For this review, take the finished solid that the model builds, in its own axes (mm). Coordinates: 2 decimals unless noted, no trailing zeros. Loops run counter-clockwise (first coordinate to the right, second up) from the corner with the lowest first, then second, coordinate; pieces in that order, holes last. Notation, with made-up numbers: (33.25, -39) - (90.25, -39) arc R18 cw to (90.25, -28) - close; hole circle Ø10 at (79, 58). An arc over 180 degrees is marked (long way). Answer as a JSON object with one key per item and string values. Group by question number.
Item 1: To check wall thickness, follow line 1 (X direction, y = 1.55, z = -45); line 2 (X direction, y = 1.4, z = 15); line 3 (Z direction, x = -20, y = 0.65). State the ranges of each line that lie inside material, in increasing order.
Item 2: Clearance check with a flat-ended pin moving along its axis: pin 1 (1.5 mm diameter, centred on y = 2.5, z = -92.5, fed in from +X). State where the tip first meets the part, or that it passes through.
Item 3: We need section B-B (z = -15). Give the boundary of the cut face in (x, y).
Item 4: We need section A-A (z = -45). Give the boundary of the cut face in (x, y), then the cut area to 3 significant figures.
Item 5: We need section D-D (y = 0.45). State how many separate pieces and enclosed holes the cut face has, then the cut area to 3 significant figures.
Item 6: We need section C-C (x = -26.5). Give the boundary of the cut face in (y, z).
Item 7: Mouldability with a two-part tool opening along X and no side actions: class faces 1 (the flat face through (-1, 0, -31)), 2 (the cylindrical face through (48.831, 1.521, 14.474)), 3 (the cylindrical face through (1.319, 1.479, -119.985)), 4 (the cylindrical face through (-57.15, 1.52, 56.99)) as released by +X, released by -X, zero draft, split by the parting line, or undercut.
from build123d import *

# Parameters (mm, degrees)
BOSS_EXTRUDE3_DEPTH = 3
FILLET3_R           = 10
SKETCH4_R           = 1.75
CUT_EXTRUDE1_DEPTH  = 3
CUT_EXTRUDE2_REACH  = 5
SKETCH5_R           = 1.75
CUT_EXTRUDE3_REACH  = 5
SKETCH6_R           = 1.5


with BuildPart() as part:
    # Sketch1 → Boss-Extrude3 (new body)
    with BuildSketch(Plane(origin=(0, 0, 0), x_dir=(1, 0, 0), z_dir=(0, 1, 0))):
        with BuildLine():
            Line((-60, 60), (-60, -60))
            Line((-60, -60), (60, -60))
            Line((60, -60), (60, 60))
            ThreePointArc((60, 60), (0, 120), (-60, 60))
        make_face()
    extrude(amount=BOSS_EXTRUDE3_DEPTH)

    # Fillet3
    fillet3_edges = [part.edges().sort_by_distance(p)[0] for p in [
        (60, 1.5, 60),
        (-60, 1.5, 60),
    ]]
    fillet(fillet3_edges, radius=FILLET3_R)

    # Sketch4 → Cut-Extrude1 (cut)
    with BuildSketch(Plane(origin=(0, 3, 0), x_dir=(1, 0, 0), z_dir=(0, 1, 0))):
        with Locations((-26.5, -15)):
            Circle(SKETCH4_R)
        with Locations((-50.5, -15)):
            Circle(SKETCH4_R)
        with Locations((-50.5, 15)):
            Circle(SKETCH4_R)
        with Locations((-26.5, 15)):
            Circle(SKETCH4_R)
    cut_extrude1 = extrude(amount=-CUT_EXTRUDE1_DEPTH, mode=Mode.SUBTRACT)

    # Mirror1: Cut-Extrude1 across plane
    add(cut_extrude1.mirror(Plane(origin=(0, 0, 0), x_dir=(0, 0, 1), z_dir=(1, 0, 0))), mode=Mode.SUBTRACT)

    # Sketch5 → Cut-Extrude2 (cut, up to next)
    with BuildSketch(Plane(origin=(0, 3, 0), x_dir=(1, 0, 0), z_dir=(0, 1, 0)), mode=Mode.PRIVATE) as cut_extrude2_sk1:
        with Locations((20, 75)):
            Circle(SKETCH5_R)
    cut_extrude2_tool1 = extrude(cut_extrude2_sk1.sketch, amount=-CUT_EXTRUDE2_REACH, mode=Mode.PRIVATE) & part.part
    add(cut_extrude2_tool1.solids().sort_by_distance((20, 3, -75))[0], mode=Mode.SUBTRACT)
    # Sketch5 → Cut-Extrude2 (cut, up to next)
    with BuildSketch(Plane(origin=(0, 3, 0), x_dir=(1, 0, 0), z_dir=(0, 1, 0)), mode=Mode.PRIVATE) as cut_extrude2_sk2:
        with Locations((-20, 75)):
            Circle(SKETCH5_R)
    cut_extrude2_tool2 = extrude(cut_extrude2_sk2.sketch, amount=-CUT_EXTRUDE2_REACH, mode=Mode.PRIVATE) & part.part
    add(cut_extrude2_tool2.solids().sort_by_distance((-20, 3, -75))[0], mode=Mode.SUBTRACT)
    # Sketch5 → Cut-Extrude2 (cut, up to next)
    with BuildSketch(Plane(origin=(0, 3, 0), x_dir=(1, 0, 0), z_dir=(0, 1, 0)), mode=Mode.PRIVATE) as cut_extrude2_sk3:
        with Locations((-20, 45)):
            Circle(SKETCH5_R)
    cut_extrude2_tool3 = extrude(cut_extrude2_sk3.sketch, amount=-CUT_EXTRUDE2_REACH, mode=Mode.PRIVATE) & part.part
    add(cut_extrude2_tool3.solids().sort_by_distance((-20, 3, -45))[0], mode=Mode.SUBTRACT)
    # Sketch5 → Cut-Extrude2 (cut, up to next)
    with BuildSketch(Plane(origin=(0, 3, 0), x_dir=(1, 0, 0), z_dir=(0, 1, 0)), mode=Mode.PRIVATE) as cut_extrude2_sk4:
        with Locations((20, 45)):
            Circle(SKETCH5_R)
    cut_extrude2_tool4 = extrude(cut_extrude2_sk4.sketch, amount=-CUT_EXTRUDE2_REACH, mode=Mode.PRIVATE) & part.part
    add(cut_extrude2_tool4.solids().sort_by_distance((20, 3, -45))[0], mode=Mode.SUBTRACT)

    # Sketch6 → Cut-Extrude3 (cut, up to next)
    with BuildSketch(Plane(origin=(0, 3, 0), x_dir=(1, 0, 0), z_dir=(0, 1, 0)), mode=Mode.PRIVATE) as cut_extrude3_sk1:
        with Locations((-38.213203436, 75.786796564)):
            Circle(SKETCH6_R)
    cut_extrude3_tool1 = extrude(cut_extrude3_sk1.sketch, amount=-CUT_EXTRUDE3_REACH, mode=Mode.PRIVATE) & part.part
    add(cut_extrude3_tool1.solids().sort_by_distance((-38.213203, 3, -75.786797))[0], mode=Mode.SUBTRACT)
    # Sketch6 → Cut-Extrude3 (cut, up to next)
    with BuildSketch(Plane(origin=(0, 3, 0), x_dir=(1, 0, 0), z_dir=(0, 1, 0)), mode=Mode.PRIVATE) as cut_extrude3_sk2:
        with Locations((-17, 97)):
            Circle(SKETCH6_R)
    cut_extrude3_tool2 = extrude(cut_extrude3_sk2.sketch, amount=-CUT_EXTRUDE3_REACH, mode=Mode.PRIVATE) & part.part
    add(cut_extrude3_tool2.solids().sort_by_distance((-17, 3, -97))[0], mode=Mode.SUBTRACT)
    # Sketch6 → Cut-Extrude3 (cut, up to next)
    with BuildSketch(Plane(origin=(0, 3, 0), x_dir=(1, 0, 0), z_dir=(0, 1, 0)), mode=Mode.PRIVATE) as cut_extrude3_sk3:
        with Locations((17, 97)):
            Circle(SKETCH6_R)
    cut_extrude3_tool3 = extrude(cut_extrude3_sk3.sketch, amount=-CUT_EXTRUDE3_REACH, mode=Mode.PRIVATE) & part.part
    add(cut_extrude3_tool3.solids().sort_by_distance((17, 3, -97))[0], mode=Mode.SUBTRACT)
    # Sketch6 → Cut-Extrude3 (cut, up to next)
    with BuildSketch(Plane(origin=(0, 3, 0), x_dir=(1, 0, 0), z_dir=(0, 1, 0)), mode=Mode.PRIVATE) as cut_extrude3_sk4:
        with Locations((38.213203436, 75.786796564)):
            Circle(SKETCH6_R)
    cut_extrude3_tool4 = extrude(cut_extrude3_sk4.sketch, amount=-CUT_EXTRUDE3_REACH, mode=Mode.PRIVATE) & part.part
    add(cut_extrude3_tool4.solids().sort_by_distance((38.213203, 3, -75.786797))[0], mode=Mode.SUBTRACT)


solid = part.part
Check sheet entries:
{
 "1": {"line 1": "x = -60 to -21.75, -18.25 to 18.25, 21.75 to 60", "line 2": "x = -60 to -52.25, -48.75 to -28.25, -24.75 to 24.75, 28.25 to 48.75, 52.25 to 60", "line 3": "z = -116.57 to -76.75, -73.25 to -46.75, -43.25 to 60"},
 "2": {"pin 1": "stops at x = 50.91"},
 "3": {"outline": "(-60, 0) - (-52.25, 0) - (-52.25, 3) - (-60, 3) - close; (-48.75, 0) - (-28.25, 0) - (-28.25, 3) - (-48.75, 3) - close; (-24.75, 0) - (24.75, 0) - (24.75, 3) - (-24.75, 3) - close; (28.25, 0) - (48.75, 0) - (48.75, 3) - (28.25, 3) - close; (52.25, 0) - (60, 0) - (60, 3) - (52.25, 3) - close"},
 "4": {"outline": "(-60, 0) - (-21.75, 0) - (-21.75, 3) - (-60, 3) - close; (-18.25, 0) - (18.25, 0) - (18.25, 3) - (-18.25, 3) - close; (21.75, 0) - (60, 0) - (60, 3) - (21.75, 3) - close", "area": "339 mm2"},
 "5": {"separate pieces": "1", "enclosed holes": "16", "area": "19,900 mm2"},
 "6": {"outline": "(0, -113.83) - (3, -113.83) - (3, -16.75) - (0, -16.75) - close; (0, -13.25) - (3, -13.25) - (3, 13.25) - (0, 13.25) - close; (0, 16.75) - (3, 16.75) - (3, 60) - (0, 60) - close"},
 "7": {"face 1": "zero draft", "face 2": "undercut", "face 3": "split by the parting line", "face 4": "released by -X"}
}
